The model under review builds one solid part; all positions refer to its coordinate system, in mm. Face numbers are marked on the shaded views. A direction names the side the tool comes from. Coordinates: 2 decimals unless noted, no trailing zeros. Write each loop counter-clockwise with the first axis right and the second up, starting at its lowest first coordinate (ties: lowest second). Pieces come first, ordered by that corner, then holes. Notation, with made-up numbers: (64.25, -35) - (97.25, -35) arc R17 ccw to (97.25, -12) - close; hole circle Ø10 at (22.5, 56.5). An arc over 180 degrees is marked (long way). Use one line per item in the form item = value. Start each with the question number.
```python
from build123d import *

# Parameters (mm, degrees)
SKETCH_1_R      = 14
SKETCH_1_R_2    = 12.25
EXTRUDE_1_DEPTH = 5
EXTRUDE_2_DEPTH = 4
SKETCH_3_R      = 15
SKETCH_3_R_2    = 13.5
EXTRUDE_3_DEPTH = 5
FILLET_2_R      = 1
FILLET_3_R      = 1
SKETCH_4_R      = 13.5
SKETCH_4_R_2    = 11
EXTRUDE_4_DEPTH = 1
FILLET_5_R      = 1


with BuildPart() as part:
    # 草图1 → 凸台-拉伸1 (new body)
    with BuildSketch(Plane(origin=(0, 0, 0), x_dir=(1, 0, 0), z_dir=(0, 1, 0))):
        with Locations(Location((0, 0, 0), (0, 0, 270))):
            Circle(SKETCH_1_R)
        with Locations(Location((0, 0, 0), (0, 0, 270))):
            Circle(SKETCH_1_R_2, mode=Mode.SUBTRACT)
    extrude(amount=EXTRUDE_1_DEPTH)

    # 草图2 → 凸台-拉伸2 (add)
    with BuildSketch(Plane(origin=(0, 0, 0), x_dir=(1, 0, 0), z_dir=(0, 1, 0))):
        with BuildLine():
            Line((-11, 5.390964663), (-11, -5.390964663))
            ThreePointArc((-11, -5.390964663), (-12.25, 0), (-11, 5.390964663))
        make_face()
        with BuildLine():
            Line((11, 5.390964663), (11, -5.390964663))
            ThreePointArc((11, -5.390964663), (12.25, 0), (11, 5.390964663))
        make_face()
    extrude(amount=EXTRUDE_2_DEPTH)

    # 草图3 → 凸台-拉伸3 (add)
    with BuildSketch(Plane(origin=(0, 0, 0), x_dir=(1, 0, 0), z_dir=(0, 1, 0))):
        with Locations(Location((0, 0, 0), (0, 0, 270))):
            Circle(SKETCH_3_R)
        with Locations(Location((0, 0, 0), (0, 0, 270))):
            Circle(SKETCH_3_R_2, mode=Mode.SUBTRACT)
    extrude(amount=-EXTRUDE_3_DEPTH)

    # 圆角2
    fillet_2_edges = [part.edges().sort_by_distance(p)[0] for p in [
        (0, 0, -14),
    ]]
    fillet(fillet_2_edges, radius=FILLET_2_R - 0.0001)  # a hair under: the kernel refuses the full size

    # 圆角3
    fillet_3_edges = [part.edges().sort_by_distance(p)[0] for p in [
        (0, 0, -15),
    ]]
    fillet(fillet_3_edges, radius=FILLET_3_R)

    # 草图4 → 凸台-拉伸4 (add)
    with BuildSketch(Plane.XZ):
        with Locations(Location((0, 0, 0), (0, 0, 90))):
            Circle(SKETCH_4_R)
        Circle(SKETCH_4_R_2, mode=Mode.SUBTRACT)
    extrude(amount=EXTRUDE_4_DEPTH)

    # 圆角5
    fillet_5_edges = [part.edges().sort_by_distance(p)[0] for p in [
        (0, -5, -13.5),
    ]]
    fillet(fillet_5_edges, radius=FILLET_5_R)


solid = part.part
```
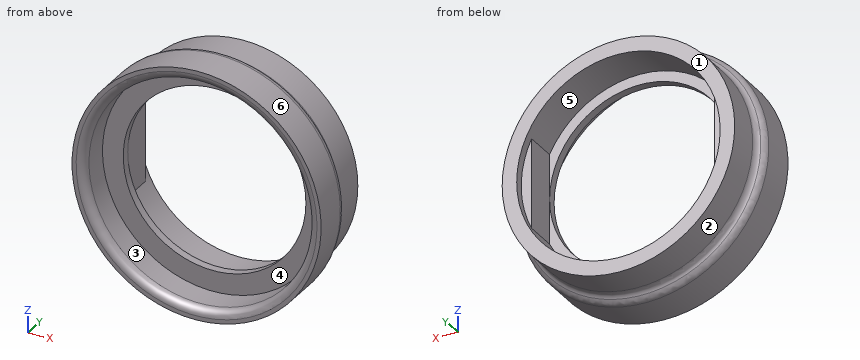
1. For the marked faces 4, 5 and 6, list the 3-axis set-ups (+Z, -Z, +X, -X, +Y, -Y) from which the entire face can be reached by the end or side of a thin tool; tool diameter is ignored.
2. For L1, parallel to Z at x = 0, y = -2.85; L2, parallel to X at y = 3.1, z = 0, list the stretches that pass through material, from the lowest coordinate up.
3. Take a section at A-A (y = 1.75). State the section outline as (x, z) points, plus the area to 3 significant figures.
4. The part is to be moulded in two halves that separate along Z. For the marked faces 1, 2 and 3, say which applies: released by +Z, released by -Z, zero draft, split by the parting line, or undercut.
5. Take a section at B-B (y = -2.25). State the section outline as (x, z) points.
6. For P1, Ø1, axis at y = 3, z = 2, coming from the -X side; P2, Ø3, axis at x = 12, y = 3.5, coming from the -Z side; P3, Ø13.5, axis at x = -0.5, z = 0, coming from the -Y side; P4, Ø3, axis at y = 1.5, z = -1, coming from the +X side, all flat-tipped, find the tip position at first contact; note any pin that passes through.
Returned:
q1.face_4 = -Y
q1.face_5 = +Y
q1.face_6 = +Y, -Y
q2.L1 = -15 to -13.5, 13.5 to 15
q2.L2 = -14 to -11, 11 to 14
q3.outline = circle Ø28 at (0, 0); hole (-11, -5.39) arc R12.25 ccw to (11, -5.39) - (11, 5.39) arc R12.25 ccw to (-11, 5.39) - close
q3.area = 162 mm²
q4.face_1 = zero draft
q4.face_2 = split by the parting line
q4.face_3 = undercut
q5.outline = circle Ø30 at (0, 0); hole circle Ø27 at (0, 0)
q6.P1 = -13.92
q6.P2 = -9.26
q6.P3 = through
q6.P4 = 14.65
